```python
from build123d import *

# Parameters (mm, degrees)
SKETCH1_W           = 70
SKETCH1_H           = 35
BOSS_EXTRUDE1_DEPTH = 32
SKETCH2_R           = 4
CUT_EXTRUDE1_DEPTH  = 40
CHAMFER1_SIZE       = 25
SKETCH3_W           = 70
SKETCH3_H           = 7
BOSS_EXTRUDE2_DEPTH = 47
SKETCH4_W           = 70
SKETCH4_H           = 3
BOSS_EXTRUDE3_DEPTH = 47
SKETCH6_R           = 1.5
CUT_EXTRUDE3_DEPTH  = 10
CHAMFER2_SIZE       = 45


with BuildPart() as part:
    # Sketch1 → Boss-Extrude1 (new body)
    with BuildSketch(Plane(origin=(0, 0, 0), x_dir=(1, 0, 0), z_dir=(0, 1, 0))):
        Rectangle(SKETCH1_W, SKETCH1_H)
    extrude(amount=BOSS_EXTRUDE1_DEPTH)

    # Sketch2 → Cut-Extrude1 (cut)
    with BuildSketch(Plane.XY.offset(17.5)):
        with Locations((0, 25)):
            Circle(SKETCH2_R)
    extrude(amount=-CUT_EXTRUDE1_DEPTH, mode=Mode.SUBTRACT)

    # Chamfer1
    chamfer1_edges = [part.edges().sort_by_distance(p)[0] for p in [
        (-35, 32, 0),
        (35, 32, 0),
    ]]
    chamfer(chamfer1_edges, length=CHAMFER1_SIZE)

    # Sketch3 → Boss-Extrude2 (add)
    with BuildSketch(Plane.XY.offset(17.5)):
        with Locations((0, 3.5)):
            Rectangle(SKETCH3_W, SKETCH3_H)
    extrude(amount=BOSS_EXTRUDE2_DEPTH)

    # Sketch4 → Boss-Extrude3 (add)
    with BuildSketch(Plane(origin=(0, 7, 0), x_dir=(1, 0, 0), z_dir=(0, 1, 0))):
        with Locations((0, -63)):
            Rectangle(SKETCH4_W, SKETCH4_H)
    extrude(amount=BOSS_EXTRUDE3_DEPTH)

    # Sketch6 → Cut-Extrude3 (cut)
    with BuildSketch(Plane.XY.offset(64.5)):
        with Locations((-27, 12.9)):
            Circle(SKETCH6_R)
        with Locations((-27, 43.5)):
            Circle(SKETCH6_R)
    extrude(amount=-CUT_EXTRUDE3_DEPTH, mode=Mode.SUBTRACT)

    # Chamfer2
    chamfer2_edges = [part.edges().sort_by_distance(p)[0] for p in [
        (35, 54, 63),
    ]]
    chamfer(chamfer2_edges, length=CHAMFER2_SIZE)


solid = part.part
```
Model file for the job. Use its own axes, mm. A direction names the side the tool comes from. Coordinates: 2 decimals unless noted, no trailing zeros. Order: outer loops, then holes, each group sorted by start corner. A loop starts at its lowest first (then second) coordinate and runs counter-clockwise, first axis right, second up. Notation, with made-up numbers: (21.5, 6.5) -> (71.5, 6.5) arc R9 ccw to (71.5, 18.5) -> close; hole circle Ø5 at (39, 44). An arc over 180 degrees is marked (long way). Answer as a JSON object with one key per item and string values. Group by question number.
1) Cut at D-D, the plane z = -4.5. Write the cut outline in (x, y).
2) Drill centre lines: L1, parallel to Y at x = -27, z = 63.4; L2, parallel to Y at x = 0, z = 3.5; L3, parallel to Z at x = 7, y = 14. Where is each one in solid material? Low to high.
3) Cut at A-A, the plane y = 15.5. Write the cut outline in (x, z).
4) Which spindle directions (+Z, -Z, +X, -X, +Y, -Y) get a long thin tool onto all of the face, cutting with end or side? Do faces 1 (the face through (-8, 25, 61.5)), 2 (the face through (23, 19, 0)), 3 (the face through (-28.5, 12.97, 63.02)). Say none if no direction does.
5) Pull direction X, two halves, no side cores. Call faces 4 (the face through (-23, 54, 63)), 5 (the face through (-0.521, 28.966, 0.245)), 6 (the face through (-22, 20, 0)): +X half, -X half, draft (parallel to the pull), parting line (faces both ways), or undercut.
6) Cut at C-C, the plane y = 25. Write the cut outline in (x, z).
7) Cut at B-B, the plane x = 0. Write the cut outline in (y, z), then the cut area to 3 significant figures.
8) Flat gauge pins, fed straight in: pin 1 (1 mm diameter, centred on x = -15.5, y = 32.5, fed in from -Z); pin 2 (1 mm diameter, centred on x = -9, z = 23, fed in from +Y); pin 3 (6 mm diameter, centred on x = -2, z = -3, fed in from +Y). Where does each tip first touch, or does it go through?
Check values:
{
 "1": {"outline": "(-35, 0) -> (35, 0) -> (35, 7) -> (10, 32) -> (-10, 32) -> (-35, 7) -> close; hole circle Ø8 at (0, 25)"},
 "2": {"L1": "y = 0 to 11.4, 14.4 to 42, 45 to 54", "L2": "y = 0 to 21, 29 to 32", "L3": "z = -17.5 to 17.5, 61.5 to 64.5"},
 "3": {"outline": "(-35, 61.5) -> (28.5, 61.5) -> (28.5, 64.5) -> (-35, 64.5) -> close; (-26.5, -17.5) -> (26.5, -17.5) -> (26.5, 17.5) -> (-26.5, 17.5) -> close"},
 "4": {"face 1": "+X, -X, +Y", "face 2": "-Z, +X, +Y", "face 3": "+Z"},
 "5": {"face 4": "draft", "face 5": "undercut", "face 6": "-X half"},
 "6": {"outline": "(-35, 61.5) -> (19, 61.5) -> (19, 64.5) -> (-35, 64.5) -> close; (-17, -17.5) -> (-4, -17.5) -> (-4, 17.5) -> (-17, 17.5) -> close; (4, -17.5) -> (17, -17.5) -> (17, 17.5) -> (4, 17.5) -> close"},
 "7": {"outline": "(0, -17.5) -> (21, -17.5) -> (21, 17.5) -> (7, 17.5) -> (7, 61.5) -> (44, 61.5) -> (44, 64.5) -> (0, 64.5) -> close; (29, -17.5) -> (32, -17.5) -> (32, 17.5) -> (29, 17.5) -> close", "area": "1,280 mm²"},
 "8": {"pin 1": "stops at z = 61.5", "pin 2": "stops at y = 7", "pin 3": "stops at y = 32"}
}
